Can you work these out from the drawing? Everything is in mm from the part's minimum corner. Coordinates: 2 decimals unless noted, no trailing zeros. Write each loop counter-clockwise with the first axis right and the second up, starting at its lowest first coordinate (ties: lowest second). Pieces come first, ordered by that corner, then holes.
(1) For pin 1 Ø4 at (x, y) = (6, 9) entering from -Z; pin 2 Ø2 at (x, z) = (9, 4.5) entering from -Y, each with a flat end and sliding along its axis, tell me the tip position at first contact or that it passes through.
(2) Imagine slicing it at C-C, the plane z = 1.75. List the corners of the cut face in (x, y) for me.
(3) Imagine slicing it at A-A, the plane y = 6.9. List the corners of the cut face in (x, z) for me.
(4) Thinking about a two-plate mould opening in X: for the marked faces 1, 2 and 3, which applies, released by +X, released by -X, zero draft, split by the parting line, or undercut?
(5) Imagine slicing it at B-B, the plane x = 8.4. List the corners of the cut face in (y, z) for me.
(6) Please list where these lines run through material, in increasing order: probe 1 along Y at (x, z) = (8.4, 4.05); probe 2 along X at (y, z) = (8.25, 1.2); probe 3 along X at (y, z) = (4, 2.15).
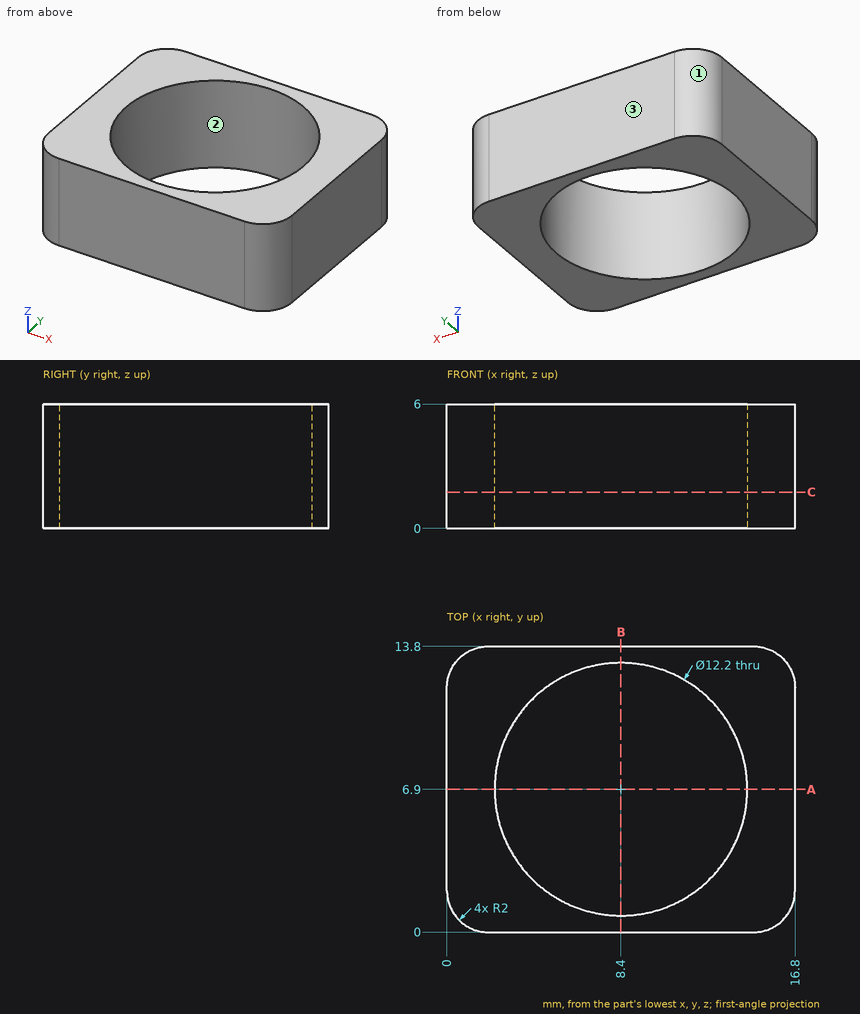
Recorded:
1. pin 1: passes through
1. pin 2: stops at y = 0
2. outline: (0, 2) arc R2 ccw to (2, 0) - (14.8, 0) arc R2 ccw to (16.8, 2) - (16.8, 11.8) arc R2 ccw to (14.8, 13.8) - (2, 13.8) arc R2 ccw to (0, 11.8) - close; hole circle Ø12.2 at (8.4, 6.9)
3. outline: (0, 0) - (2.3, 0) - (2.3, 6) - (0, 6) - close; (14.5, 0) - (16.8, 0) - (16.8, 6) - (14.5, 6) - close
4. face 1: released by -X
4. face 2: undercut
4. face 3: zero draft
5. outline: (0, 0) - (0.8, 0) - (0.8, 6) - (0, 6) - close; (13, 0) - (13.8, 0) - (13.8, 6) - (13, 6) - close
6. probe 1: y = 0 to 0.8, 13 to 13.8
6. probe 2: x = 0 to 2.45, 14.35 to 16.8
6. probe 3: x = 0 to 3.03, 13.77 to 16.8
